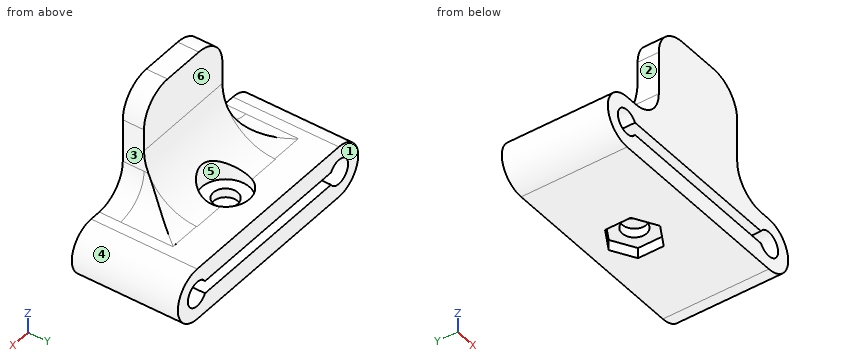
```python
from build123d import *

# Parameters (mm, degrees)
SKETCH_1_R               = 1.175
EXTRUDE_1_DEPTH          = 10
SKETCH_3_W               = 10
SKETCH_3_H               = 15
EXTRUDE_2_DEPTH          = 2
FILLET_2_R               = 3
FILLET_START             = -5
FILLET_3_DEPTH           = 10
FILLET_START_2           = 2
FILLET_3_2_DEPTH         = 4.9438
FILLET_START_3           = -9
FILLET_3_3_DEPTH         = 17
SKETCH_4_W               = 16.05948
SKETCH_4_H               = 1.2
CUT_EXTRUDE_2_DEPTH      = 20.735795
CUT_EXTRUDE_4_DEPTH      = 19.271738
CUT_EXTRUDE_4_DEPTH_BACK = 1
SKETCH_6_R               = 2.25
SKETCH_7_R               = 1.15
CUT_EXTRUDE_5_DEPTH      = 19.841879
CUT_EXTRUDE_6_DEPTH      = 1


with BuildPart() as part:
    # 草图1 → 凸台-拉伸1 (new body)
    with BuildSketch(Plane(origin=(0, 0, 0), x_dir=(1, 0, 0), z_dir=(0, 1, 0))):
        with BuildLine():
            Line((-9.04, 2.46), (9.04, 2.46))
            ThreePointArc((9.04, 2.46), (11.5, 0), (9.04, -2.46))
            Line((9.04, -2.46), (-9.04, -2.46))
            ThreePointArc((-9.04, -2.46), (-11.5, 0), (-9.04, 2.46))
        make_face()
        with Locations(Location((9.04, 0, 0), (0, 0, 270))):
            Circle(SKETCH_1_R, mode=Mode.SUBTRACT)
        with Locations(Location((-9.04, 0, 0), (0, 0, 90))):
            Circle(SKETCH_1_R, mode=Mode.SUBTRACT)
    extrude(amount=EXTRUDE_1_DEPTH)

    # 草图3 → 凸台-拉伸2 (add)
    with BuildSketch(Plane.XZ):
        with Locations((0, 5.04)):
            Rectangle(SKETCH_3_W, SKETCH_3_H)
    extrude(amount=-EXTRUDE_2_DEPTH)

    # 圆角2
    fillet_2_edges = [part.edges().sort_by_distance(p)[0] for p in [
        (5, 1, 12.54),
        (5, 1, 2.46),
        (-5, 1, 2.46),
        (-5, 1, 12.54),
    ]]
    fillet(fillet_2_edges, radius=FILLET_2_R)

    # 圆角3: read off the stored shape, not the designer's step
    # 圆角3 outline → 圆角3 (add)
    with BuildSketch(Plane.YZ.offset(FILLET_START)):
        with BuildLine():
            ThreePointArc((7, 2.46), (3.464466, 3.924466), (2, 7.46))
            Line((2, 7.46), (2, 2.46))
            Line((2, 2.46), (7, 2.46))
        make_face()
    extrude(amount=FILLET_3_DEPTH)

    # Fillet 3 2 outline → Fillet 3 2 (add)
    with BuildSketch(Plane(origin=(0, 0, 0), x_dir=(1, 0, 0), z_dir=(0, 1, 0)).offset(FILLET_START_2)):
        with BuildLine():
            Line((5, -2.46), (5, -5.46))
            ThreePointArc((5, -5.46), (5.87868, -3.33868), (8, -2.46))
            Line((8, -2.46), (5, -2.46))
        make_face()
        with BuildLine():
            Line((-5, -5.46), (-5, -2.46))
            Line((-5, -2.46), (-8, -2.46))
            ThreePointArc((-8, -2.46), (-5.87868, -3.33868), (-5, -5.46))
        make_face()
    extrude(amount=FILLET_3_2_DEPTH)

    # Fillet 3 3 outline → Fillet 3 3 (cut)
    with BuildSketch(Plane.YZ.offset(FILLET_START_3)):
        with BuildLine():
            Line((8, 7), (2.021205, 7))
            ThreePointArc((2.021205, 7), (3.610313, 3.784402), (6.9438, 2.460316))
            ThreePointArc((6.9438, 2.460316), (6.9719, 2.460079), (7, 2.46))
            Line((7, 2.46), (8, 2.46))
            Line((8, 2.46), (8, 7))
        make_face()
    extrude(amount=FILLET_3_3_DEPTH, mode=Mode.SUBTRACT)

    # 草图4 → 切除-拉伸2 (cut, through all)
    with BuildSketch(Plane.XZ):
        Rectangle(SKETCH_4_W, SKETCH_4_H)
    extrude(amount=-CUT_EXTRUDE_2_DEPTH, mode=Mode.SUBTRACT)

    # 草图6 → 切除-拉伸4 (cut, two sides: drawn at the far end of the back side and taken through both)
    with BuildSketch(Plane.XY.offset(2.46).offset(-CUT_EXTRUDE_4_DEPTH_BACK)):
        with Locations(Location((0, 6, 0), (0, 0, 153.6122))):
            Circle(SKETCH_6_R)
    extrude(amount=CUT_EXTRUDE_4_DEPTH + CUT_EXTRUDE_4_DEPTH_BACK, mode=Mode.SUBTRACT)

    # 草图7 → 切除-拉伸5 (cut, through all)
    with BuildSketch(Plane.XY.offset(1.46)):
        with Locations((0, 6)):
            Circle(SKETCH_7_R)
    extrude(amount=-CUT_EXTRUDE_5_DEPTH, mode=Mode.SUBTRACT)

    # 草图8 → 切除-拉伸6 (cut)
    with BuildSketch(Plane(origin=(0, 0, -2.46), x_dir=(-1, 0, 0), z_dir=(0, 0, -1))):
        Polygon((0, 8.424871), (-2.1, 7.212436), (-2.1, 4.787564), (0, 3.575129), (2.1, 4.787564), (2.1, 7.212436), align=None)
    extrude(amount=-CUT_EXTRUDE_6_DEPTH, mode=Mode.SUBTRACT)


solid = part.part
```
Verification items for the finished model (mm, model axes). Face numbers are marked on the shaded views. A direction names the side the tool comes from. Coordinates: 2 decimals unless noted, no trailing zeros. Write each loop counter-clockwise with the first axis right and the second up, starting at its lowest first coordinate (ties: lowest second). Pieces come first, ordered by that corner, then holes. Notation, with made-up numbers: (56, 48) - (74, 48) arc R32 ccw to (74, 84) - close; hole circle Ø8 at (78.25, -29.75). An arc over 180 degrees is marked (long way). One line per question, with ' | ' between items. Start each with the question number.
1. Section check D-D (y = 4.25). Enter the section's corners in (x, z) (3 decimals), plus the area to 3 significant figures.
2. Section check A-A (z = 0). Enter the section's corners in (x, y) (3 decimals).
3. Gauge pin test, flat ends, axial feed: P1, Ø2.5, axis at x = 0, y = 6, coming from the -Z side; P2, Ø2, axis at x = 0, y = 6, coming from the +Z side; P3, Ø4, axis at x = 1.5, y = 7, coming from the -Z side; P4, Ø0.8, axis at y = 6, z = -2, coming from the +X side. Record the tip position at first contact, or that the pin passes through.
4. Draft check along X on the marked faces 4, 5 and 6. Enter one of: released by +X, released by -X, zero draft, split by the parting line, or undercut.
5. Material ranges on line 1 along Z through (x, y) = (3.75, 8.5); line 2 along Y through (x, z) = (0, 1.2); line 3 along X through (y, z) = (3.5, 0) (3 decimals), recorded low to high.
6. Access from +Z, -Z, +X, -X, +Y, -Y to the whole of each face (thin tool, end or side, straight path). Record for the marked faces 1, 2 and 3.
7. Section check C-C (x = 3). Enter the section's corners in (y, z).
8. Section check B-B (y = 6). Enter the section's corners in (x, z) (3 decimals), plus the area to 3 significant figures.
Computed values:
1) outline: (-9.04, -2.46) - (-1.169, -2.46) - (-1.169, -1.46) - (1.169, -1.46) - (1.169, -2.46) - (9.04, -2.46) arc R2.46 ccw to (9.04, 2.46) - (8, 2.46) arc R3 cw to (5.935, 3.284) - (1.414, 3.284) - (1.414, 1.46) - (-1.414, 1.46) - (-1.414, 3.284) - (-5.935, 3.284) arc R3 cw to (-8, 2.46) - (-9.04, 2.46) arc R2.46 ccw to start; hole (-8.03, -0.6) - (8.03, -0.6) arc R1.175 ccw (long way) to (8.03, 0.6) - (-8.03, 0.6) arc R1.175 ccw (long way) to start | area: 83.6 mm²
2) outline: (-11.5, 0) - (-10.215, 0) - (-10.215, 10) - (-11.5, 10) - close; (10.215, 0) - (11.5, 0) - (11.5, 10) - (10.215, 10) - close
3) P1: z = -1.46 | P2: through | P3: z = -2.46 | P4: x = 10.91
4) face 4: released by +X | face 5: undercut | face 6: zero draft
5) line 1: -2.46 to -0.6, 0.6 to 2.46 | line 2: 0 to 4.85, 7.15 to 10 | line 3: -11.5 to -10.215, 10.215 to 11.5
6) face 1: +Z, -Z, +X, -X, +Y | face 2: +Z, -X, +Y, -Y | face 3: +Z, +X, +Y, -Y
7) outline: (0, -2.46) - (10, -2.46) - (10, -0.6) - (0, -0.6) - close; (0, 0.6) - (10, 0.6) - (10, 2.46) - (7, 2.46) arc R5 cw to (2, 7.46) - (2, 12.37) - (0, 12.37) - close
8) outline: (-9.04, -2.46) - (-2.1, -2.46) - (-2.1, -1.46) - (-1.15, -1.46) - (-1.15, -0.6) - (-8.03, -0.6) arc R1.175 cw (long way) to (-8.03, 0.6) - (-1.15, 0.6) - (-1.15, 1.46) - (-2.25, 1.46) - (-2.25, 2.561) - (-7.228, 2.561) arc R3 cw to (-8, 2.46) - (-9.04, 2.46) arc R2.46 ccw to start; (1.15, -1.46) - (2.1, -1.46) - (2.1, -2.46) - (9.04, -2.46) arc R2.46 ccw to (9.04, 2.46) - (8, 2.46) arc R3 cw to (7.228, 2.561) - (2.25, 2.561) - (2.25, 1.46) - (1.15, 1.46) - (1.15, 0.6) - (8.03, 0.6) arc R1.175 cw (long way) to (8.03, -0.6) - (1.15, -0.6) - close | area: 68.7 mm²
